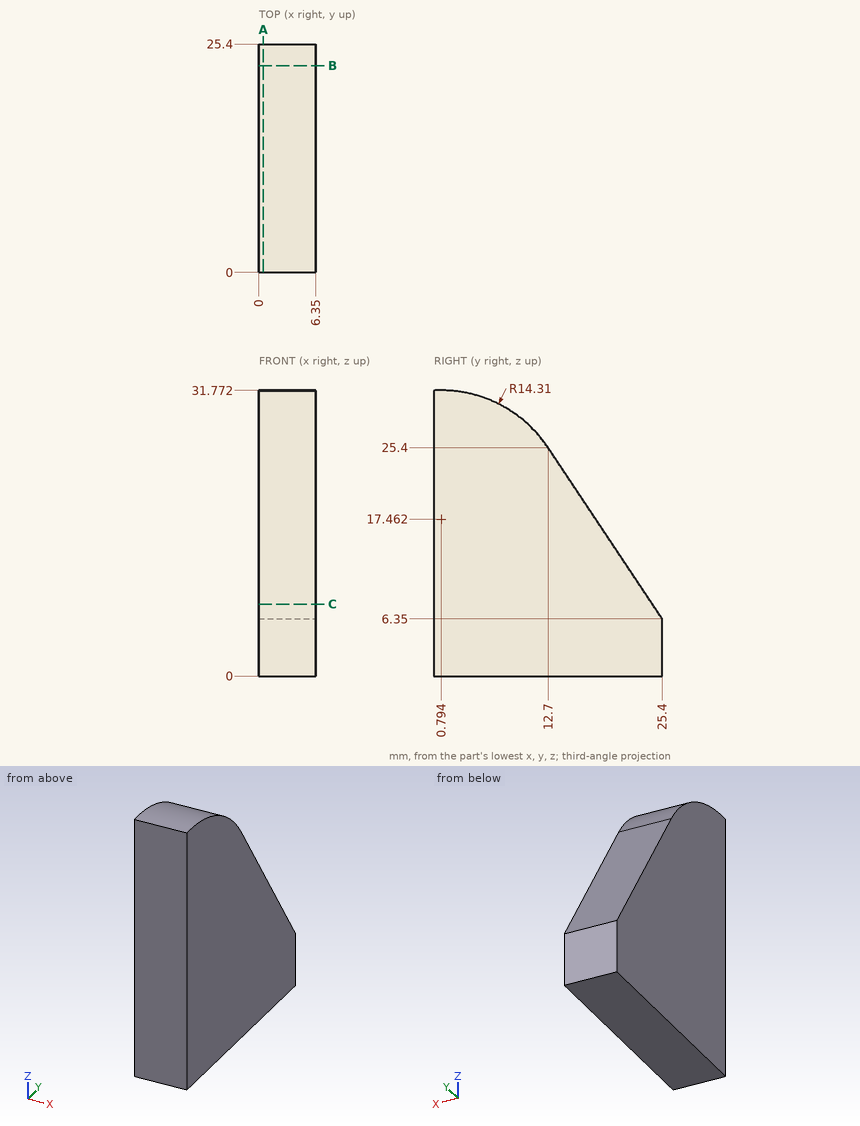
Answer from the drawing. Dimensions are ordinates in mm from the lowest x, y and z of the part. Give positions to 0.01 mm unless a question says otherwise; leave off trailing zeros. Loops run counter-clockwise (first coordinate to the right, second up) from the corner with the lowest first, then second, coordinate; pieces in that order, holes last. Notation, with made-up numbers: M -38,49.5 L 5,49.5 A17 ccw 5,56.5 Z; hole C 3,73.25 d1. An arc over 180 degrees is marked long. One line per item, written item: value.
Q1. A cutting plane is placed at A-A on x = 0.5. Determine the outline of the cut face in (y, z).
Working result:
outline: M 0,0 L 25.4,0 L 25.4,6.35 L 12.7,25.4 A14.31 ccw 0,31.75 Z
Q2. Find the intervals of material crossed by line 1 (Z direction, x = 2, y = 1); line 2 (Z direction, x = 2.5, y = 13.25) (1 decimal); line 3 (Y direction, x = 5.5, z = 13) (1 decimal), in increasing order. Write a range as from..to.
Working result:
line 1: z = 0..31.77
line 2: z = 0..24.6
line 3: y = 0..21
Q3. A cutting plane is placed at C-C on z = 8. Determine the outline of the cut face in (x, y).
Working result:
outline: M 0,0 L 6.35,0 L 6.35,24.3 L 0,24.3 Z
Q4. Flat-ended cylindrical pins translate along their axes: P1, Ø2, axis at x = 3, z = 25.5, coming from the +Y side; P2, Ø2, axis at x = 2.5, y = 5.5, coming from the +Z side. Find the tip coordinate at first contact, or state that the pin passes through.
Working result:
P1: stops at y = 13.3
P2: stops at z = 31.28
Q5. A cutting plane is placed at B-B on y = 23. Determine the outline of the cut face in (x, z).
Working result:
outline: M 0,0 L 6.35,0 L 6.35,9.95 L 0,9.95 Z
